Design review of the part built by this model. Coordinates are the model's own, in mm. Face numbers are marked on the shaded views. A direction names the side the tool comes from. Round coordinates to 2 decimals unless told otherwise and drop trailing zeros. Write each loop counter-clockwise with the first axis right and the second up, starting at its lowest first coordinate (ties: lowest second). Pieces come first, ordered by that corner, then holes. Notation, with made-up numbers: (80.25, -20.75) - (121.25, -20.75) arc R16 ccw to (121.25, -8.75) - close; hole circle Ø7 at (-14.5, 16). An arc over 180 degrees is marked (long way). Use one line per item in the form item = value.
```python
from build123d import *

# Parameters (mm, degrees)
CROQUIS2_R                 = 16.5
CROQUIS2_R_2               = 15
SALIENTE_EXTRUIR1_DEPTH    = 12
CROQUIS3_R                 = 18.5
SALIENTE_EXTRUIR2_DEPTH    = 2
CROQUIS4_R                 = 15
CORTAR_EXTRUIR1_DEPTH      = 2
CORTAR_EXTRUIR2_DEPTH      = 22
CORTAR_EXTRUIR2_DEPTH_BACK = 21
CROQUIS5_R                 = 2


with BuildPart() as part:
    # Croquis2 → Saliente-Extruir1 (new body)
    with BuildSketch(Plane.XY):
        Circle(CROQUIS2_R)
        Circle(CROQUIS2_R_2, mode=Mode.SUBTRACT)
    extrude(amount=SALIENTE_EXTRUIR1_DEPTH)

    # Croquis3 → Saliente-Extruir2 (add)
    with BuildSketch(Plane.XY.offset(12)):
        Circle(CROQUIS3_R)
    extrude(amount=-SALIENTE_EXTRUIR2_DEPTH)

    # Croquis4 → Cortar-Extruir1 (cut)
    with BuildSketch(Plane(origin=(0, 0, 10), x_dir=(-1, 0, 0), z_dir=(0, 0, -1))):
        Circle(CROQUIS4_R)
    extrude(amount=-CORTAR_EXTRUIR1_DEPTH, mode=Mode.SUBTRACT)

    # Croquis5 → Cortar-Extruir2 (cut, two sides: drawn at the far end of the back side and taken through both)
    with BuildSketch(Plane(origin=(0, 0, 0), x_dir=(1, 0, 0), z_dir=(0, 1, 0)).offset(-CORTAR_EXTRUIR2_DEPTH_BACK)):
        with Locations(Location((0, -5, 0), (0, 0, 90))):
            Circle(CROQUIS5_R)
    extrude(amount=CORTAR_EXTRUIR2_DEPTH + CORTAR_EXTRUIR2_DEPTH_BACK, mode=Mode.SUBTRACT)


solid = part.part
```
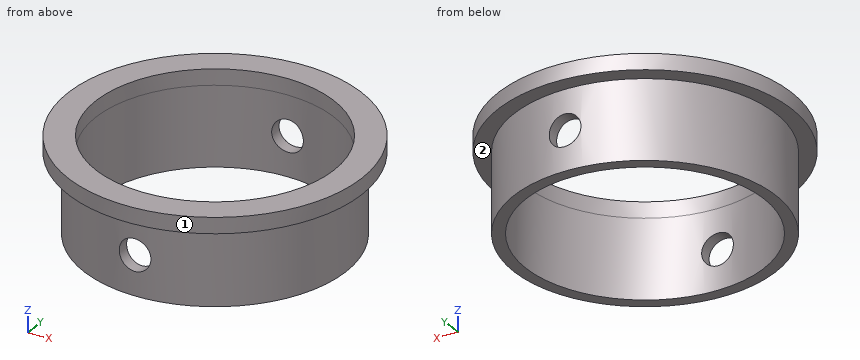
Q1. We need section B-B on x = 11. Write out the cut boundary in (y, z), then the cut area to 3 significant figures.
Calculated:
outline = (-14.87, 10) - (-12.3, 10) - (-12.3, 0) - (-10.2, 0) - (-10.2, 12) - (-14.87, 12) - close; (10.2, 0) - (12.3, 0) - (12.3, 10) - (14.87, 10) - (14.87, 12) - (10.2, 12) - close
area = 60.7 mm2
Q2. For P1, Ø5, axis at y = 13, z = 7, coming from the -X side; P2, Ø3, axis at x = 0, z = 5, coming from the +Y side (1 decimal); P3, Ø1, axis at x = -4, z = 10, coming from the -Y side; P4, Ø4.5, axis at x = 0, z = 5, coming from the -Y side, all flat-tipped, find the tip position at first contact; note any pin that passes through.
Calculated:
P1 = -12.73
P2 = through
P3 = -18.17
P4 = -16.5
Q3. Machinability: for the marked faces 1 and 2, which of the approach directions +Z, -Z, +X, -X, +Y, -Y give a long, thin tool a straight path to every point of the face, cutting with its end or side? Answer none if there is none.
Calculated:
face_1 = +Z, -Z
face_2 = -Z
Q4. We need section D-D on x = 0. Write out the cut boundary in (y, z).
Calculated:
outline = (-18.5, 10) - (-16.5, 10) - (-16.5, 7) - (-15, 7) - (-15, 12) - (-18.5, 12) - close; (-16.5, 0) - (-15, 0) - (-15, 3) - (-16.5, 3) - close; (15, 0) - (16.5, 0) - (16.5, 3) - (15, 3) - close; (15, 7) - (16.5, 7) - (16.5, 10) - (18.5, 10) - (18.5, 12) - (15, 12) - close
Q5. To check wall thickness, follow line 1 along Y through (x, z) = (0, 10.9); line 2 along X through (y, z) = (9, 6); line 3 along X through (y, z) = (2, 2.5). State the ranges of each line that lie inside material, in increasing order. Write a range as from..to.
Calculated:
line_1 = -18.5..-15, 15..18.5
line_2 = -13.83..-12, 12..13.83
line_3 = -16.38..-14.87, 14.87..16.38
Q6. We need section A-A on y = 0. Write out the cut boundary in (x, z).
Calculated:
outline = (-18.5, 10) - (-16.5, 10) - (-16.5, 0) - (-15, 0) - (-15, 12) - (-18.5, 12) - close; (15, 0) - (16.5, 0) - (16.5, 10) - (18.5, 10) - (18.5, 12) - (15, 12) - close
